Read the model definition and answer for the solid it produces. Units are mm, in the model's axes. A direction names the side the tool comes from. Coordinates: 2 decimals unless noted, no trailing zeros. Loops run counter-clockwise (first coordinate to the right, second up) from the corner with the lowest first, then second, coordinate; pieces in that order, holes last. Notation, with made-up numbers: M 51.5,30 L 106.5,30 A5 cw 106.5,36 Z; hole C 75,67 d1. An arc over 180 degrees is marked long. Put each result on its own line as item: value.
from build123d import *

# Parameters (mm, degrees)
BASE_FLANGE1_DEPTH = 201.168
CUT_EXTRUDE1_DEPTH = 10
LPATTERN1_COUNT    = 11
LPATTERN1_PITCH    = 25


# Sheet-metal steps are written as plain solids
with BuildPart() as part:
    # Sketch1 → Base-Flange1 (new body)
    with BuildSketch(Plane.XY):
        with BuildLine():
            Line((0, 0), (3.2634, 0))
            ThreePointArc((3.2634, 0), (4.491361636, -0.508638364), (5, -1.7366))
            Line((5, -1.7366), (5, -6.7634))
            ThreePointArc((5, -6.7634), (5.215745145, -7.284254855), (5.7366, -7.5))
            Line((5.7366, -7.5), (31.2634, -7.5))
            ThreePointArc((31.2634, -7.5), (31.784254855, -7.284254855), (32, -6.7634))
            Line((32, -6.7634), (32, -1.7366))
            ThreePointArc((32, -1.7366), (32.508638364, -0.508638364), (33.7366, 0))
            Line((33.7366, 0), (37, 0))
            Line((37, 0), (37, -1))
            Line((37, -1), (33.7366, -1))
            ThreePointArc((33.7366, -1), (33.215745145, -1.215745145), (33, -1.7366))
            Line((33, -1.7366), (33, -6.7634))
            ThreePointArc((33, -6.7634), (32.491361636, -7.991361636), (31.2634, -8.5))
            Line((31.2634, -8.5), (5.7366, -8.5))
            ThreePointArc((5.7366, -8.5), (4.508638364, -7.991361636), (4, -6.7634))
            Line((4, -6.7634), (4, -1.7366))
            ThreePointArc((4, -1.7366), (3.784254855, -1.215745145), (3.2634, -1))
            Line((3.2634, -1), (0, -1))
            Line((0, -1), (0, 0))
        make_face()
    extrude(amount=BASE_FLANGE1_DEPTH)

    # Sketch6 → Cut-Extrude1 (cut)
    with BuildSketch(Plane(origin=(0, -7.5, 0), x_dir=(1, 0, 0), z_dir=(0, 1, 0))):
        with BuildLine():
            Line((21.3866, -174.168), (21.3866, -188.168))
            ThreePointArc((21.3866, -188.168), (18.2366, -191.318), (15.0866, -188.168))
            Line((15.0866, -188.168), (15.0866, -174.168))
            ThreePointArc((15.0866, -174.168), (18.2366, -171.018), (21.3866, -174.168))
        make_face()
    cut_extrude1 = extrude(amount=-CUT_EXTRUDE1_DEPTH, mode=Mode.SUBTRACT)

    # LPattern1: Cut-Extrude1 ×11
    with Locations(*[(0, 0, -i * LPATTERN1_PITCH) for i in range(1, LPATTERN1_COUNT)]):
        add(cut_extrude1, mode=Mode.SUBTRACT)


solid = part.part
1) Find section C-C, the plane x = 25. Write down the section's boundary in (y, z).
Answer list:
outline: M -8.5,0 L -7.5,0 L -7.5,201.17 L -8.5,201.17 Z
2) Given pin 1 Ø0.5 at (y, z) = (-8, 128) entering from -X; pin 2 Ø1.1 at (y, z) = (-8, 181) entering from -X; pin 3 Ø0.8 at (y, z) = (-8, 80) entering from +X, each flat-ended and moving along its own axis, determine where each tip first touches the part or whether it passes through.
Answer list:
pin 1: stops at x = 4.31
pin 2: stops at x = 4.14
pin 3: stops at x = 32.79
3) Straight lines are drawn through the part: line 1 (X direction, y = -2.25, z = 174); line 2 (Y direction, x = 25.5, z = 85.5); line 3 (X direction, y = -8, z = 71.5). For each, find the intervals that lie inside material, in ascending order. Write a range as [from, to].
Answer list:
line 1: x = [4, 5], [32, 33]
line 2: y = [-8.5, -7.5]
line 3: x = [4.52, 16.56], [19.91, 32.48]
4) Find section A-A, the plane z = 85. Write down the section's boundary in (x, y), plus the area to 3 significant figures.
Answer list:
outline: M 0,-1 L 3.26,-1 A0.74 cw 4,-1.74 L 4,-6.76 A1.74 ccw 5.74,-8.5 L 15.09,-8.5 L 15.09,-7.5 L 5.74,-7.5 A0.74 cw 5,-6.76 L 5,-1.74 A1.74 ccw 3.26,0 L 0,0 Z; M 21.39,-8.5 L 31.26,-8.5 A1.74 ccw 33,-6.76 L 33,-1.74 A0.74 cw 33.74,-1 L 37,-1 L 37,0 L 33.74,0 A1.74 ccw 32,-1.74 L 32,-6.76 A0.74 cw 31.26,-7.5 L 21.39,-7.5 Z
area: 43.6 mm^2
5) Find section B-B, the plane y = -4.25. Write down the section's boundary in (x, z).
Answer list:
outline: M 4,0 L 5,0 L 5,201.17 L 4,201.17 Z; M 32,0 L 33,0 L 33,201.17 L 32,201.17 Z
6) Which of the six approach directions +Z, -Z, +X, -X, +Y, -Y give full straight-line access (tool end or side, diameter ignored) to faces 4 (the cylindrical face through (18.17, -7.99, 121.02)), 5 (the flat face through (35, -1, 99)), 6 (the flat face through (35, 0, 99)), 7 (the flat face through (19, -8, 201.168)), 8 (the flat face through (32, -4, 99))?
Answer list:
face 4: +Y, -Y
face 5: +Z, -Z, +X, -Y
face 6: +Z, -Z, +X, -X, +Y
face 7: +Z, +X, -X, +Y, -Y
face 8: +Z, -Z, +Y
7) Determine the mould class of faces 1 (the cylindrical face through (18.306, -7.993, 166.317)), 2 (the flat face through (2, -1, 99)), 3 (the flat face through (4, -4, 99)) for opening direction X: released by +X, released by -X, zero draft, split by the parting line, or undercut.
Answer list:
face 1: undercut
face 2: zero draft
face 3: released by -X
